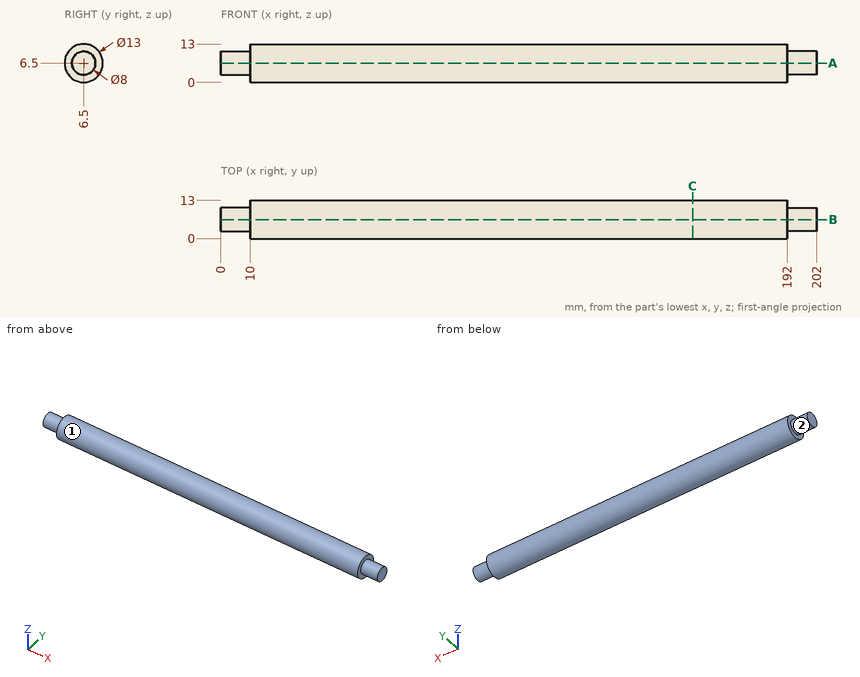
Geometry: see drawing. Coordinates: mm, zero at the bounding-box minimum. A direction names the side the tool comes from. Round coordinates to 2 decimals unless told otherwise and drop trailing zeros. Loops run counter-clockwise (first coordinate to the right, second up) from the corner with the lowest first, then second, coordinate; pieces in that order, holes last. Notation, with made-up numbers: M -39.5,48.25 L 8.5,48.25 A11 cw 8.5,54.25 Z; hole C 89.25,33 d6. An arc over 180 degrees is marked long. Use a Markdown table: item, result. Add a question column.
1. Section query C-C on x = 160. Return the cut outline in (y, z).
2. Line query: line 1 (X direction, y = 12, z = 7.25); line 2 (Z direction, x = 96, y = 7); line 3 (Y direction, x = 156, z = 6.75). Output: solid intervals per line, ascending.
3. Section query A-A on z = 6.5. Return the cut outline in (x, y), then the cut area to 3 significant figures.
4. Reachability of the marked faces 1 and 2 from +Z, -Z, +X, -X, +Y, -Y: full face, straight path, thin tool, end or side. Return the list, or none.
5. Contact query for flat-ended pins moving along their axis: P1, Ø3, axis at x = 81.5, z = 2.5, coming from the -Y side; P2, Ø4, axis at x = 100, y = 2, coming from the +Z side; P3, Ø5, axis at x = 149.5, z = 2, coming from the -Y side. Output: stop coordinate, or through.
Reported:
| question | item | result |
|---|---|---|
| 1 | outline | C 6.5,6.5 d13 |
| 2 | line 1 | x = 10 to 192 |
| 2 | line 2 | z = 0.02 to 12.98 |
| 2 | line 3 | y = 0 to 13 |
| 3 | outline | M 0,2.5 L 10,2.5 L 10,0 L 192,0 L 192,2.5 L 202,2.5 L 202,10.5 L 192,10.5 L 192,13 L 10,13 L 10,10.5 L 0,10.5 Z |
| 3 | area | 2,530 mm² |
| 4 | face 1 | +X, -X |
| 4 | face 2 | -X |
| 5 | P1 | stops at y = 0.5 |
| 5 | P2 | stops at z = 12.5 |
| 5 | P3 | stops at y = 0.32 |
